Autodesk Inventor part; units mm, degrees
ref_plane "YZ Plane" through (0, 0, 0) normal (1, 0, 0) x (0, 1, 0)
ref_plane "XZ Plane" through (0, 0, 0) normal (0, 1, 0) x (-1, 0, 0)
ref_plane "XY Plane" through (0, 0, 0) normal (0, 0, 1) x (1, 0, 0)
sketch "スケッチ1" plane through (0, 0, 0) normal (0, 0, 1) x (1, 0, 0)
  line L0 (-20, -20) -> (20, -20)
  line L1 (20, -20) -> (20, 20)
  line L2 (20, 20) -> (-20, 20)
  line L3 (-20, 20) -> (-20, -20)
  line L4 (-20, -20) -> (20, 20) construction
  line L5 (20, -20) -> (-20, 20) construction
  point P0 (0, 0)
  dimension "d0" = 40
  dimension "d1" = 40
extrude "押し出し1" add sketch "スケッチ1" along normal blind 60
sketch "スケッチ2" plane through (0, 0, 60) normal (0, 0, 1) x (1, 0, 0)
  line L0 (20, 20) -> (-20, 20)
  line L1 (10, -20) -> (-10, -20)
  line L2 (-10, -20) -> (-10, 20)
  line L3 (-10, 20) -> (10, 20)
  line L4 (10, 20) -> (10, -20)
  line L5 (10, -20) -> (-10, 20) construction
  line L6 (-10, -20) -> (10, 20) construction
  point P0 (0, 0)
  dimension "d4" = 20
extrude "押し出し2" cut sketch "スケッチ2" against normal blind 55
sketch "スケッチ4" plane through (0, 0, 60) normal (0, 0, 1) x (1, 0, 0)
  point P0 (0, 0)
  point P1 (-15, 0)
  point P2 (15, 0)
  dimension "d7" = 15
  dimension "d8" = 15
hole "穴1" at (-15, 0, 60) at (15, 0, 60) direction (0, 0, -1) diameter 3.2 depth 6 tip angle 118
sketch "スケッチ5" plane through (-20, -20, 0) normal (0, -1, 0) x (1, 0, 0)
  line L0 (0, 60) -> (10, 60)
  line L1 (30, 60) -> (40, 60)
  line L2 (3, 50) -> (37, 50)
  line L3 (3, 50) -> (3, 5)
  line L4 (3, 5) -> (37, 5)
  line L5 (37, 5) -> (37, 50)
  line L6 (0, 0) -> (0, 60)
  line L7 (40, 0) -> (40, 60)
  point P0 (20, 0)
  dimension "d16" = 10
  dimension "d17" = 10
  dimension "d20" = 3
  dimension "d21" = 3
extrude "押し出し3" cut sketch "スケッチ5" against normal blind 55
sketch "スケッチ7" plane through (0, 0, 0) normal (0, 0, -1) x (-1, 0, 0)
  point P0 (0, 0)
  point P1 (15, -5)
  point P2 (15, 5)
  point P3 (-15, 5)
  point P4 (-15, -5)
  dimension "d37" = 15
  dimension "d38" = 5
  dimension "d39" = 5
  dimension "d40" = 15
  dimension "d41" = 5
  dimension "d42" = 15
  dimension "d43" = 5
  dimension "d44" = 15
hole "穴3" at (-15, -5, 0) at (-15, 5, 0) at (15, 5, 0) at (15, -5, 0) direction (0, 0, 1) diameter 3.2 depth 8.8 tip angle 118
properties part number "20220703_Fan Fixed"
Design review of the part built by this model. Coordinates are the model's own, in mm. A direction names the side the tool comes from. Give positions to 0.01 mm unless a question says otherwise; leave off trailing zeros. Order: outer loops, then holes, each group sorted by start corner. A loop starts at its lowest first (then second) coordinate and runs counter-clockwise, first axis right, second up.
1. To check wall thickness, follow L1, parallel to X at y = -5, z = 3.2; L2, parallel to X at y = 0, z = 58.2; L3, parallel to Z at x = -16.5, y = 17.5. State the ranges of each line that lie inside material, in increasing order.
Solution:
L1: x = -20 to -16.6, -13.4 to 13.4, 16.6 to 20
L2: x = -20 to -16.6, -13.4 to -10, 10 to 13.4, 16.6 to 20
L3: z = 0 to 5, 50 to 60
2. For pin 1 Ø3 at (x, y) = (-15, -5) entering from -Z; pin 2 Ø12 at (x, z) = (6, 36) entering from +Y; pin 3 Ø1 at (x, y) = (6, 12.5) entering from +Z; pin 4 Ø2.5 at (x, y) = (15, 0) entering from +Z, all flat-tipped, find the tip position at first contact; note any pin that passes through.
Solution:
pin 1: stops at z = 50
pin 2: passes through
pin 3: stops at z = 5
pin 4: stops at z = 53.79
3. Add section A-A, the plane z = 23. State the section outline as (x, y) points.
Solution:
outline: (-20, -20) - (-17, -20) - (-17, 20) - (-20, 20) - close; (17, -20) - (20, -20) - (20, 20) - (17, 20) - close
4. Add section D-D, the plane x = 4.5. State the section outline as (y, z) points, then the cut area to 3 significant figures.
Solution:
outline: (-20, 0) - (20, 0) - (20, 5) - (-20, 5) - close
area: 200 mm2
5. Add section C-C, the plane y = -2.5. State the section outline as (x, z) points.
Solution:
outline: (-20, 0) - (20, 0) - (20, 60) - (10, 60) - (10, 50) - (17, 50) - (17, 5) - (-17, 5) - (-17, 50) - (-10, 50) - (-10, 60) - (-20, 60) - close
6. Add section B-B, the plane y = 5. State the section outline as (x, z) points, then the cut area to 3 significant figures.
Solution:
outline: (-20, 0) - (-16.6, 0) - (-16.6, 5) - (-17, 5) - (-17, 50) - (-10, 50) - (-10, 60) - (-20, 60) - close; (-13.4, 0) - (13.4, 0) - (13.4, 5) - (-13.4, 5) - close; (10, 50) - (17, 50) - (17, 5) - (16.6, 5) - (16.6, 0) - (20, 0) - (20, 60) - (10, 60) - close
area: 638 mm2
7. Mouldability with a two-part tool opening along Y and no side actions: class faces 1 (the flat face through (17, 0, 27)), 2 (the conical face through (14.729, 0.06, 53.206)), 3 (the flat face through (18, 20, 28)) as +Y half, -Y half, draft (parallel to the pull), parting line (faces both ways), or undercut.
Solution:
face 1: draft
face 2: undercut
face 3: +Y half
8. Tool access review of faces 4 (the cylindrical face through (13.92, -6.18, 2.54)), 5 (the flat face through (0, 0, 5)), 6 (the cylindrical face through (13.414, 0.208, 56.958)): name each direction out of +Z, -Z, +X, -X, +Y, -Y from which nothing blocks a thin tool from reaching the whole face with its end or side.
Solution:
face 4: -Z
face 5: +Y, -Y
face 6: +Z
